Can you work these out from the model? Positions are in its coordinate system, mm. Face numbers are marked on the shaded views. A direction names the side the tool comes from. Give positions to 0.01 mm unless a question says otherwise; leave off trailing zeros. Loops run counter-clockwise (first coordinate to the right, second up) from the corner with the lowest first, then second, coordinate; pieces in that order, holes last. Notation, with made-up numbers: (84, 52.25) -> (90, 52.25) arc R26 cw to (90, 83.25) -> close; hole circle Ø6 at (45.25, 78). An arc over 180 degrees is marked (long way). Return JSON: item names as keys, results as strings. Group by question number.
Q1. Suppose I cut it at D-D, the plane z = -2. Please give me the cut outline in (x, y), and give its area (4 significant figures).
Q2. Which directions (+Z, -Z, +X, -X, +Y, -Y) give clear straight access to the entire face, cutting with the end or side of a thin tool? Please do the marked faces 1, 2 and 3.
Q3. Suppose I cut it at C-C, the plane z = 0.75. Please give me the cut outline in (x, y), and give its area (3 significant figures).
Q4. I need wall thicknesses on line 1 along X through (y, z) = (3.75, -0.5); line 2 along Z through (x, y) = (8.5, 9); line 3 along X through (y, z) = (6.5, 0). Which ranges of each line are inside material? Lowest first, please. Write a range as [from, to].
Q5. Suppose I cut it at A-A, the plane y = 2.25. Please give me the cut outline in (x, z), and give its area (3 significant figures).
Q6. Will these pins go through, and if not, where does the flat tip stop? pin 1 (1 mm diameter, centred on x = 3, z = -1, fed in from -Y); pin 2 (1.8 mm diameter, centred on x = -8.5, z = 0, fed in from -Y).
Q7. Thinking about a two-plate mould opening in X: for the marked faces 4, 5 and 6, which applies, pulls with the +X half, pulls with the -X half, needs draft (parallel to the pull), parting line crosses it, or undercut?
Q8. Suppose I cut it at B-B, the plane x = -8.5. Please give me the cut outline in (y, z), and give its area (3 significant figures).
```python
from build123d import *

# Parameters (mm, degrees)
SKETCH1_W           = 20
SKETCH1_H           = 6
SKETCH1_R           = 1
BOSS_EXTRUDE1_DEPTH = 3
SKETCH2_W           = 13
SKETCH2_H           = 6
CUT_EXTRUDE1_DEPTH  = 1.25
CHAMFER1_SIZE       = 2
SKETCH3_R           = 1.5
SKETCH3_R_2         = 1
BOSS_EXTRUDE2_DEPTH = 7.5


with BuildPart() as part:
    # Sketch1 → Boss-Extrude1 (new body)
    with BuildSketch(Plane(origin=(0, 0, 0), x_dir=(1, 0, 0), z_dir=(0, 1, 0))):
        Rectangle(SKETCH1_W, SKETCH1_H)
        with Locations((-8.5, 0)):
            Circle(SKETCH1_R, mode=Mode.SUBTRACT)
        with Locations((8.5, 0)):
            Circle(SKETCH1_R, mode=Mode.SUBTRACT)
    extrude(amount=BOSS_EXTRUDE1_DEPTH)

    # Sketch2 → Cut-Extrude1 (cut)
    with BuildSketch(Plane(origin=(0, 3, 0), x_dir=(1, 0, 0), z_dir=(0, 1, 0))):
        Rectangle(SKETCH2_W, SKETCH2_H)
    extrude(amount=-CUT_EXTRUDE1_DEPTH, mode=Mode.SUBTRACT)

    # Chamfer1
    chamfer1_edges = [part.edges().sort_by_distance(p)[0] for p in [
        (10, 1.5, 3),
        (-10, 1.5, 3),
        (-10, 1.5, -3),
        (10, 1.5, -3),
    ]]
    chamfer(chamfer1_edges, length=CHAMFER1_SIZE)

    # Sketch3 → Boss-Extrude2 (add)
    with BuildSketch(Plane(origin=(0, 3, 0), x_dir=(1, 0, 0), z_dir=(0, 1, 0))):
        with Locations((-8.5, 0)):
            Circle(SKETCH3_R)
        with Locations((-8.5, 0)):
            Circle(SKETCH3_R_2, mode=Mode.SUBTRACT)
    boss_extrude2 = extrude(amount=BOSS_EXTRUDE2_DEPTH)

    # Mirror1: Boss-Extrude2 across plane
    add(boss_extrude2.mirror(Plane(origin=(0, 0, 0), x_dir=(0, 0, 1), z_dir=(1, 0, 0))))


solid = part.part
```
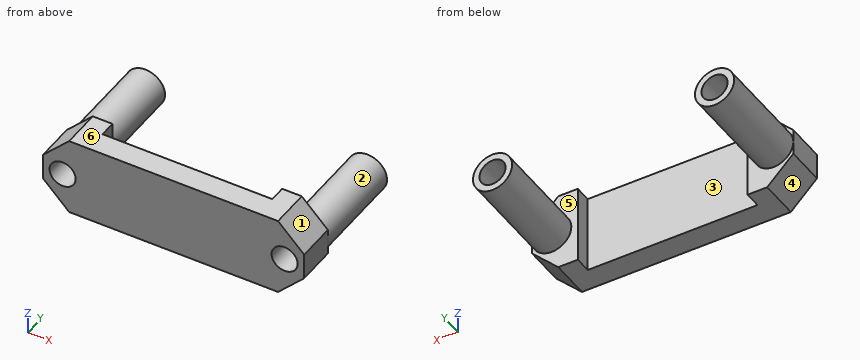
Ans:
{
 "1": {"outline": "(-9, 0) -> (9, 0) -> (9, 3) -> (6.5, 3) -> (6.5, 1.75) -> (-6.5, 1.75) -> (-6.5, 3) -> (-9, 3) -> close", "area": "37.75 mm^2"},
 "2": {"face 1": "+Z, +X, +Y, -Y", "face 2": "+Y", "face 3": "+Z, -Z, +Y"},
 "3": {"outline": "(-10, 0) -> (-9.16, 0) -> (-9.16, 10.5) -> (-9.8, 10.5) -> (-9.8, 3) -> (-10, 3) -> close; (-7.84, 0) -> (7.84, 0) -> (7.84, 10.5) -> (7.2, 10.5) -> (7.2, 3) -> (6.5, 3) -> (6.5, 1.75) -> (-6.5, 1.75) -> (-6.5, 3) -> (-7.2, 3) -> (-7.2, 10.5) -> (-7.84, 10.5) -> close; (9.16, 0) -> (10, 0) -> (10, 3) -> (9.8, 3) -> (9.8, 10.5) -> (9.16, 10.5) -> close", "area": "54.9 mm^2"},
 "4": {"line 1": "x = [-9.91, -9.37], [-7.63, -7.09], [7.09, 7.63], [9.37, 9.91]", "line 2": "z = [-1.5, -1], [1, 1.5]", "line 3": "x = [-10, -9.5], [-7.5, -7], [7, 7.5], [9.5, 10]"},
 "5": {"outline": "(-10, -1) -> (-8, -3) -> (-6.5, -3) -> (-6.5, 3) -> (-8, 3) -> (-10, 1) -> close; (6.5, -3) -> (8, -3) -> (10, -1) -> (10, 1) -> (8, 3) -> (6.5, 3) -> close; hole circle Ø2 at (-8.5, 0); hole circle Ø2 at (8.5, 0)", "area": "27.7 mm^2"},
 "6": {"pin 1": "stops at y = 0", "pin 2": "passes through"},
 "7": {"face 4": "pulls with the -X half", "face 5": "undercut", "face 6": "needs draft"},
 "8": {"outline": "(0, -2.5) -> (3, -2.5) -> (3, -1.5) -> (10.5, -1.5) -> (10.5, -1) -> (0, -1) -> close; (0, 1) -> (10.5, 1) -> (10.5, 1.5) -> (3, 1.5) -> (3, 2.5) -> (0, 2.5) -> close", "area": "16.5 mm^2"}
}
